Check sheet for the modelled part. Datum: model origin and axes. Units: mm. A direction names the side the tool comes from. Coordinates: 2 decimals unless noted, no trailing zeros. Loops run counter-clockwise (first coordinate to the right, second up) from the corner with the lowest first, then second, coordinate; pieces in that order, holes last. Notation, with made-up numbers: (88.5, 16.5) - (99.5, 16.5) arc R26 ccw to (99.5, 43.5) - close; hole circle Ø6 at (45, -28.5). An arc over 180 degrees is marked (long way). Answer as a JSON object with one key per item and string values. Group by question number.
from build123d import *

# Parameters (mm, degrees)
SKETCH1_R           = 4.5
BOSS_EXTRUDE3_DEPTH = 38
CUT_EXTRUDE2_DEPTH  = 1.5
CUT_EXTRUDE3_DEPTH  = 7.5
SKETCH6_W           = 7.945575041
SKETCH6_H           = 4
CUT_EXTRUDE4_DEPTH  = 26


with BuildPart() as part:
    # Sketch1 → Boss-Extrude3 (new body)
    with BuildSketch(Plane.XY):
        with Locations((-11.304886055, 8.134003381)):
            Circle(SKETCH1_R)
    extrude(amount=BOSS_EXTRUDE3_DEPTH)

    # Sketch3 → Cut-Extrude2 (cut)
    with BuildSketch(Plane.XY):
        with BuildLine():
            Line((-13.304886055, 9.634003381), (-9.304886055, 9.634003381))
            ThreePointArc((-9.304886055, 9.634003381), (-11.304886055, 10.634003381), (-13.304886055, 9.634003381))
        make_face()
        with BuildLine():
            Line((-9.304886055, 6.634003381), (-13.304886055, 6.634003381))
            ThreePointArc((-13.304886055, 6.634003381), (-11.304886055, 5.634003381), (-9.304886055, 6.634003381))
        make_face()
    extrude(amount=CUT_EXTRUDE2_DEPTH, mode=Mode.SUBTRACT)

    # Sketch3<4> → Cut-Extrude3 (cut)
    with BuildSketch(Plane.XY):
        with BuildLine():
            ThreePointArc((-8.804886055, 8.134003381), (-8.93317781, 8.924572796), (-9.304886055, 9.634003381))
            Line((-9.304886055, 9.634003381), (-13.304886055, 9.634003381))
            ThreePointArc((-13.304886055, 9.634003381), (-13.804886055, 8.134003381), (-13.304886055, 6.634003381))
            Line((-13.304886055, 6.634003381), (-9.304886055, 6.634003381))
            ThreePointArc((-9.304886055, 6.634003381), (-8.93317781, 7.343433966), (-8.804886055, 8.134003381))
        make_face()
    extrude(amount=CUT_EXTRUDE3_DEPTH, mode=Mode.SUBTRACT)

    # Sketch6 → Cut-Extrude4 (cut)
    with BuildSketch(Plane.XY.offset(38)):
        with Locations((-7.332098535, 8.134003381)):
            Rectangle(SKETCH6_W, SKETCH6_H)
    extrude(amount=-CUT_EXTRUDE4_DEPTH, mode=Mode.SUBTRACT)


solid = part.part
1. Sectioned sample at B-B on x = -12. Record the cut outline in (y, z).
2. Sectioned sample at C-C on z = 3.5. Record the cut outline in (x, y), plus the area to 3 significant figures.
3. Sectioned sample at D-D on z = 16.5. Record the cut outline in (x, y).
4. Material ranges on line 1 (X direction, y = 8.25, z = 29); line 2 (Z direction, x = -12.5, y = 10.25); line 3 (Y direction, x = -13.5, z = 2.5), recorded low to high.
5. Access from +Z, -Z, +X, -X, +Y, -Y to the whole of each face (thin tool, end or side, straight path). Record for faces 5 (the face through (-13, 8, 38)), 6 (the face through (-11, 6.634, 4)), 7 (the face through (-9, 10.134, 25)).
6. Sectioned sample at A-A on y = 9. Record the cut outline in (x, z).
7. Gauge pin test, flat ends, axial feed: pin 1 (0.5 mm diameter, centred on x = -11.5, y = 6, fed in from -Z); pin 2 (2 mm diameter, centred on x = -10.5, z = 33, fed in from +Y); pin 3 (1.2 mm diameter, centred on x = -9.5, z = 20.5, fed in from -Y); pin 4 (3 mm diameter, centred on x = -9.5, y = 8.5, fed in from +Z). Record the tip position at first contact, or that the pin passes through.
8. Release check for a two-part mould opening along X. For faces 1 (the face through (-11.305, 8, 25)), 2 (the face through (-9, 6.134, 25)), 3 (the face through (-11, 10, 1.5)), 4 (the face through (-15.8, 8.3, 18.7)) record: released by +X, released by -X, zero draft, split by the parting line, or undercut.
Answers follow:
{
 "1": {"outline": "(3.69, 0) - (5.73, 0) - (5.73, 1.5) - (6.63, 1.5) - (6.63, 7.5) - (9.63, 7.5) - (9.63, 1.5) - (10.54, 1.5) - (10.54, 0) - (12.58, 0) - (12.58, 38) - (3.69, 38) - close"},
 "2": {"outline": "circle Ø9 at (-11.3, 8.13); hole (-13.3, 6.63) - (-9.3, 6.63) arc R2.5 ccw to (-9.3, 9.63) - (-13.3, 9.63) arc R2.5 ccw to start", "area": "49.6 mm^2"},
 "3": {"outline": "(-11.3, 6.13) - (-11.3, 10.13) - (-7.27, 10.13) arc R4.5 ccw (long way) to (-7.27, 6.13) - close"},
 "4": {"line 1": "x = -15.8 to -11.3", "line 2": "z = 1.5 to 38", "line 3": "y = 4.21 to 6.94, 9.33 to 12.06"},
 "5": {"face 5": "+Z, +X, -X, +Y, -Y", "face 6": "-Z", "face 7": "+Z, +X"},
 "6": {"outline": "(-15.72, 0) - (-13.65, 0) - (-13.65, 7.5) - (-8.96, 7.5) - (-8.96, 0) - (-6.89, 0) - (-6.89, 12) - (-11.3, 12) - (-11.3, 38) - (-15.72, 38) - close"},
 "7": {"pin 1": "stops at z = 1.5", "pin 2": "stops at y = 12.63", "pin 3": "stops at y = 3.8", "pin 4": "stops at z = 12"},
 "8": {"face 1": "released by +X", "face 2": "zero draft", "face 3": "undercut", "face 4": "split by the parting line"}
}
